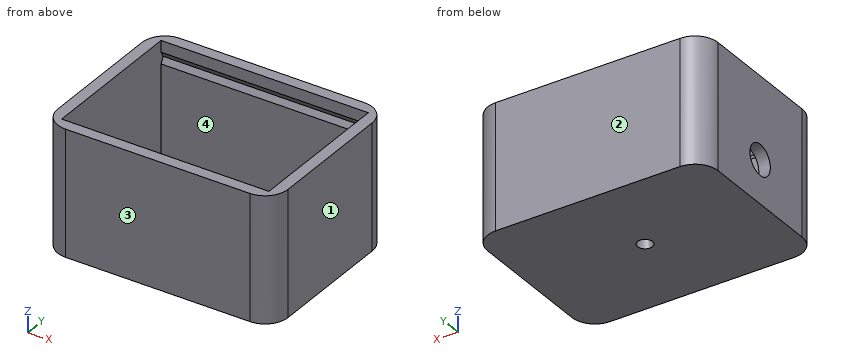
from build123d import *

# Parameters (mm, degrees)
F0_W          = 50.8
F0_H          = 38.1
F1_DEPTH      = 2.286
F2_W          = 50.8
F2_H          = 38.1
F2_W_2        = 45.72
F2_H_2        = 33.02
F3_DEPTH      = 25.4
F6_DEPTH      = 12.7
F6_DEPTH_BACK = 33.02
F8_D          = 3.3
F10_D         = 6.7564
F10_DEPTH     = 38.1
F10_TIP       = 2.0298273432
F11_R         = 5.08


with BuildPart() as f1:
    # F0 (on Top) → F1 (new body)
    with BuildSketch(Plane.XY):
        with Locations((25.4, 19.05)):
            Rectangle(F0_W, F0_H)
    extrude(amount=F1_DEPTH)

    # F2 (on face) → F3 (join)
    with BuildSketch(Plane.XY.offset(2.286)):
        with Locations((25.4, 19.05)):
            Rectangle(F2_W, F2_H)
        with Locations((25.4, 19.05)):
            Rectangle(F2_W_2, F2_H_2, mode=Mode.SUBTRACT)
    extrude(amount=F3_DEPTH)

    # F5 (on offset) → F6 (cut, two sides)
    with BuildSketch(Plane.YZ.offset(15.24)) as f6_sk:
        Polygon((2.54, 22.606), (2.54, 25.146), (1.8067651581, 23.876), align=None)
        Polygon((36.2932348419, 23.876), (35.56, 25.146), (35.56, 22.606), align=None)
    extrude(amount=-F6_DEPTH, mode=Mode.SUBTRACT)
    extrude(f6_sk.sketch, amount=F6_DEPTH_BACK, mode=Mode.SUBTRACT)

    # F8 (through all)
    with Locations(Plane.XY.offset(2.286)):
        with Locations((25.4, 19.05)):
            Hole(F8_D / 2)

    # F10
    with Locations(Plane(origin=(0, 0, 0), x_dir=(0, -1, 0), z_dir=(-1, 0, 0))):
        with Locations((-19.05, 9.525)):
            Hole(F10_D / 2, depth=F10_DEPTH)
            with Locations((0, 0, -(F10_DEPTH + F10_TIP / 2))):  # 118° drill point
                Cone(0, F10_D / 2, F10_TIP, mode=Mode.SUBTRACT)

    # F11
    f11_edges = [f1.edges().sort_by_distance(p)[0] for p in [
        (0, 0, 13.843),
        (50.8, 0, 13.843),
        (50.8, 38.1, 13.843),
        (0, 38.1, 13.843),
    ]]
    fillet(f11_edges, radius=F11_R)


solid = f1.part
Input: part model. Units: mm. Frame: model coordinates. Face numbers are marked on the shaded views. Give positions to 0.01 mm unless a question says otherwise; leave off trailing zeros. Loops run counter-clockwise (first coordinate to the right, second up) from the corner with the lowest first, then second, coordinate; pieces in that order, holes last. Notation, with made-up numbers: M 34.25,-10 L 65.25,-10 A14 ccw 65.25,14 Z; hole C 81,-37 d6. An arc over 180 degrees is marked long. Use CSV: the item, a comma, the result in double quotes.
(1) Pin query (flat end, axial travel): P1, Ø2, axis at x = 38.5, y = 27, coming from the +Z side. Return the tip coordinate at first contact, or that it passes through.
Outcome:
P1,"stops at z = 2.29"
(2) Section C-C, the plane y = 19.05. Return loops of the section in (x, z).
Outcome:
outline,"M 0,0 L 23.75,0 L 23.75,2.29 L 2.54,2.29 L 2.54,6.15 L 0,6.15 Z; M 0,12.9 L 2.54,12.9 L 2.54,27.69 L 0,27.69 Z; M 27.05,0 L 50.8,0 L 50.8,27.69 L 48.26,27.69 L 48.26,2.29 L 27.05,2.29 Z"
(3) Material intervals for L1, parallel to Y at x = 13.5, z = 7.75; L2, parallel to X at y = 30.5, z = 19.75; L3, parallel to Z at x = 1.05, y = 19.05, sorted ascending. Write a range as [from, to].
Outcome:
L1,"y = [0, 2.54], [35.56, 38.1]"
L2,"x = [0, 2.54], [48.26, 50.8]"
L3,"z = [0, 6.15], [12.9, 27.69]"
(4) Pull-direction query (Y, two-part tool) for the marked faces 1, 2, 3 and 4; classes: pulls with the +Y half, pulls with the -Y half, needs draft (parallel to the pull), parting line crosses it, or undercut.
Outcome:
face 1,"needs draft"
face 2,"pulls with the +Y half"
face 3,"pulls with the -Y half"
face 4,"undercut"
(5) Section B-B, the plane x = 25.4. Return loops of the section in (y, z), plus the area to 3 significant figures.
Outcome:
outline,"M 0,0 L 17.4,0 L 17.4,2.29 L 2.54,2.29 L 2.54,22.61 L 1.81,23.88 L 2.54,25.15 L 2.54,27.69 L 0,27.69 Z; M 20.7,0 L 38.1,0 L 38.1,27.69 L 35.56,27.69 L 35.56,25.15 L 36.29,23.88 L 35.56,22.61 L 35.56,2.29 L 20.7,2.29 Z"
area,"207 mm²"
(6) Section A-A, the plane z = 16. Return loops of the section in (x, y).
Outcome:
outline,"M 0,5.08 A5.08 ccw 5.08,0 L 45.72,0 A5.08 ccw 50.8,5.08 L 50.8,33.02 A5.08 ccw 45.72,38.1 L 5.08,38.1 A5.08 ccw 0,33.02 Z; hole M 2.54,2.54 L 48.26,2.54 L 48.26,35.56 L 2.54,35.56 Z"
(7) Section D-D, the plane z = 11. Return loops of the section in (x, y).
Outcome:
outline,"M 0,5.08 A5.08 ccw 5.08,0 L 45.72,0 A5.08 ccw 50.8,5.08 L 50.8,33.02 A5.08 ccw 45.72,38.1 L 5.08,38.1 A5.08 ccw 0,33.02 L 0,22.09 L 2.54,22.09 L 2.54,35.56 L 48.26,35.56 L 48.26,2.54 L 2.54,2.54 L 2.54,16.01 L 0,16.01 Z"
